```python
from build123d import *

# Parameters (mm, degrees)
SKETCH1_R           = 25
BOSS_EXTRUDE2_DEPTH = 10
BOSS_EXTRUDE3_DEPTH = 10
SKETCH4_R           = 3
CUT_EXTRUDE2_DEPTH  = 97.5
SKETCH5_W           = 3
SKETCH5_H           = 5.436144239
CUT_EXTRUDE3_DEPTH  = 97.5


with BuildPart() as part:
    # Sketch1 → Boss-Extrude2 (new, symmetric)
    with BuildSketch(Plane.XY):
        Circle(SKETCH1_R)
    extrude(amount=BOSS_EXTRUDE2_DEPTH, both=True)

    # Sketch1_3 → Boss-Extrude3 (add, symmetric)
    # profile 1 of 2: a face of its own
    with BuildSketch(Plane.XY):
        with BuildLine():
            Line((7.884503622, 98.138756352), (0, 100))
            Line((0, 100), (0, 89.888889442))
            Line((0, 89.888889442), (11.213955839, 72.921079468))
            ThreePointArc((11.213955839, 72.921079468), (12.316550373, 70.691845049), (12.834937175, 68.259464338))
            Line((12.834937175, 68.259464338), (13.800806716, 56.964350292))
            ThreePointArc((13.800806716, 56.964350292), (13.669977908, 54.291385078), (12.834937175, 51.748833961))
            Line((12.834937175, 51.748833961), (6.940860801, 39.594948009))
            Line((6.940860801, 39.594948009), (-4.426865135, 24.604935787))
            ThreePointArc((-4.426865135, 24.604935787), (4.287847937, 24.629542425), (12.48152348, 21.661292012))
            Line((12.48152348, 21.661292012), (21.497992968, 37.309091643))
            ThreePointArc((21.497992968, 37.309091643), (26.841650785, 58.585915514), (20.205597304, 79.495738735))
            Line((20.205597304, 79.495738735), (7.884503622, 98.138756352))
        make_face()
        Polygon((19.533386731, 37.745734284), (6.940860801, 33.450581193), (12.834937175, 42.472237729), align=None, mode=Mode.SUBTRACT)
        Polygon((3.83716906, 87.415069014), (3.83716906, 93.802296931), (9.5460666, 87.415069014), align=None, mode=Mode.SUBTRACT)
        Polygon((9.5460666, 82.8271631), (12.834937175, 85.766752133), (11.213955839, 77.937246944), align=None, mode=Mode.SUBTRACT)
        Polygon((20.448297379, 44.680987458), (12.834937175, 46.61922619), (19.533386731, 56.112338166), align=None, mode=Mode.SUBTRACT)
        Polygon((13.800806716, 72.921079468), (18.439962301, 79.495738735), (19.474189612, 66.57358604), align=None, mode=Mode.SUBTRACT)
        Polygon((23.968839315, 59.187642414), (16.637498164, 64.038154232), (23.968839315, 64.038154232), align=None, mode=Mode.SUBTRACT)
    # profile 2 of 2: a face of its own
    with BuildSketch(Plane.XY):
        with BuildLine():
            Line((-6.940860801, -39.594948009), (4.426865135, -24.604935787))
            ThreePointArc((4.426865135, -24.604935787), (-4.287847937, -24.629542425), (-12.48152348, -21.661292012))
            Line((-12.48152348, -21.661292012), (-21.497992968, -37.309091643))
            ThreePointArc((-21.497992968, -37.309091643), (-26.841650785, -58.585915514), (-20.205597304, -79.495738735))
            Line((-20.205597304, -79.495738735), (-7.884503622, -98.138756352))
            Line((-7.884503622, -98.138756352), (0, -100))
            Line((0, -100), (0, -89.888889442))
            Line((0, -89.888889442), (-11.213955839, -72.921079468))
            ThreePointArc((-11.213955839, -72.921079468), (-12.316550373, -70.691845049), (-12.834937175, -68.259464338))
            Line((-12.834937175, -68.259464338), (-13.800806716, -56.964350292))
            ThreePointArc((-13.800806716, -56.964350292), (-13.669977908, -54.291385078), (-12.834937175, -51.748833961))
            Line((-12.834937175, -51.748833961), (-6.940860801, -39.594948009))
        make_face()
        Polygon((-23.968839315, -59.187642414), (-16.637498164, -64.038154232), (-23.968839315, -64.038154232), align=None, mode=Mode.SUBTRACT)
        Polygon((-13.800806716, -72.921079468), (-18.439962301, -79.495738735), (-19.474189612, -66.57358604), align=None, mode=Mode.SUBTRACT)
        Polygon((-20.448297379, -44.680987458), (-12.834937175, -46.61922619), (-19.533386731, -56.112338166), align=None, mode=Mode.SUBTRACT)
        Polygon((-9.5460666, -82.8271631), (-12.834937175, -85.766752133), (-11.213955839, -77.937246944), align=None, mode=Mode.SUBTRACT)
        Polygon((-3.83716906, -87.415069014), (-3.83716906, -93.802296931), (-9.5460666, -87.415069014), align=None, mode=Mode.SUBTRACT)
        Polygon((-19.533386731, -37.745734284), (-6.940860801, -33.450581193), (-12.834937175, -42.472237729), align=None, mode=Mode.SUBTRACT)
    extrude(amount=BOSS_EXTRUDE3_DEPTH, both=True)

    # Sketch4 → Cut-Extrude2 (cut, symmetric)
    with BuildSketch(Plane(origin=(0, 0, -10), x_dir=(-1, 0, 0), z_dir=(0, 0, -1))):
        with Locations(Location((0, 0, 0), (0, 0, 180))):
            Circle(SKETCH4_R)
    extrude(amount=CUT_EXTRUDE2_DEPTH, both=True, mode=Mode.SUBTRACT)

    # Sketch5 → Cut-Extrude3 (cut, symmetric)
    with BuildSketch(Plane(origin=(0, 0, -10), x_dir=(-1, 0, 0), z_dir=(0, 0, -1))):
        with Locations((0, 1.280154418)):
            Rectangle(SKETCH5_W, SKETCH5_H)
    extrude(amount=CUT_EXTRUDE3_DEPTH, both=True, mode=Mode.SUBTRACT)


solid = part.part
```
Source: CAD feature listing. Evaluate the final solid. Frame: model axes, mm. A direction names the side the tool comes from. Round coordinates to 2 decimals unless told otherwise and drop trailing zeros. Loops run counter-clockwise (first coordinate to the right, second up) from the corner with the lowest first, then second, coordinate; pieces in that order, holes last. Notation, with made-up numbers: M 5,17.25 L 22,17.25 A18 ccw 22,52.25 Z; hole C 85,-27 d11. An arc over 180 degrees is marked long. Use a Markdown table: item, result. Add a question column.
1. Cut plane A-A, the plane y = 0. Output: boundary loops of the cut face in (x, z), and give its area (3 significant figures).
2. Pull-direction query (Y, two-part tool) for faces 4 (the cylindrical face through (12.305, 70.725, -0.14)), 5 (the flat face through (-14.13, -88.69, 0.14)), 6 (the flat face through (3.997, 99.056, -0.14)); classes: +Y half, -Y half, draft (parallel to the pull), parting line (faces both ways), or undercut.
3. Cut plane C-C, the plane y = -62. Output: boundary loops of the cut face in (x, z).
4. Cut plane B-B, the plane z = -1.75. State how many separate pieces and enclosed holes the cut face has, and give its area (3 significant figures).
5. Set-up query: faces 1 (the flat face through (-13.31, -62.69, 0.14)), 2 (the flat face through (1.337, 32.205, -0.14)), 3 (the flat face through (-4, 0, 10)). Return all of +Z, -Z, +X, -X, +Y, -Y with unobstructed straight access to the full face (end or side cutting, diameter ignored); none if empty.
6. Contact query for flat-ended pins moving along their axis: pin 1 (8 mm diameter, centred on x = -21, z = -3.5, fed in from +Y); pin 2 (4.5 mm diameter, centred on x = 7, z = -4, fed in from +Y); pin 3 (1.9 mm diameter, centred on y = -90, z = 2.5, fed in from -X). Output: stop coordinate, or through.
7. Ray query, line 1 along X through (y, z) = (0, -0.5); line 2 along Y through (x, z) = (17, -3.5) (3 decimals); line 3 along Y through (x, z) = (-14, 7.25). Return the intervals inside material, ascending. Write a range as [from, to].
Solution:
| question | item | result |
|---|---|---|
| 1 | outline | M -25,-10 L -3,-10 L -3,10 L -25,10 Z; M 3,-10 L 25,-10 L 25,10 L 3,10 Z |
| 1 | area | 880 mm2 |
| 2 | face 4 | undercut |
| 2 | face 5 | -Y half |
| 2 | face 6 | +Y half |
| 3 | outline | M -26.59,-10 L -23.97,-10 L -23.97,10 L -26.59,10 Z; M -19.72,-10 L -13.37,-10 L -13.37,10 L -19.72,10 Z |
| 4 | separate pieces | 1 |
| 4 | enclosed holes | 13 |
| 4 | area | 3,690 mm2 |
| 5 | face 1 | +Z, -Z, +X |
| 5 | face 2 | +Z, -Z, -X |
| 5 | face 3 | +Z, +X, -X, +Y, -Y |
| 6 | pin 1 | stops at y = 18.33 |
| 6 | pin 2 | stops at y = 98.88 |
| 6 | pin 3 | stops at x = -13.89 |
| 7 | line 1 | x = [-25, -3], [3, 25] |
| 7 | line 2 | y = [-18.33, 18.33], [29.503, 36.882], [39.533, 45.559], [52.522, 63.798], [64.038, 69.342], [77.455, 84.346] |
| 7 | line 3 | y = [-88.89, -73.2], [-72.7, -48.27], [-46.32, -41.65], [-35.86, -24.3], [-20.71, 20.71] |
